from build123d import *

# Parameters (mm, degrees)
MODEL_R             = 4.950133
MODEL_R_2           = 1.45002
MODEL_R_3           = 1.45
MODEL_R_4           = 1.5
MODEL_W             = 4
MODEL_H             = 3
MODEL_W_2           = 21.736231
MODEL_W_3           = 3
MODEL_H_2           = 2
MODEL_W_4           = 2
MODEL_H_3           = 5
BOSS_EXTRUDE1_DEPTH = 3


with BuildPart() as part:
    # Model → Boss-Extrude1 (new body)
    with BuildSketch(Plane.XY):
        with BuildLine():
            Line((330.563429791, 166.163919592), (330.563429791, 120.063919592))
            Line((330.563429791, 120.063919592), (328.431544791, 120.063919592))
            Line((328.431544791, 120.063919592), (328.431544791, 117.063919592))
            Line((328.431544791, 117.063919592), (325.431544791, 117.063919592))
            Line((325.431544791, 117.063919592), (325.431544791, 120.063919592))
            Line((325.431544791, 120.063919592), (271.695313791, 120.063919592))
            Line((271.695313791, 120.063919592), (271.695313791, 117.063919592))
            Line((271.695313791, 117.063919592), (268.695313791, 117.063919592))
            Line((268.695313791, 117.063919592), (268.695313791, 120.063919592))
            Line((268.695313791, 120.063919592), (266.463429791, 120.063919592))
            Line((266.463429791, 120.063919592), (266.463429791, 122.295819592))
            Line((266.463429791, 122.295819592), (263.463429791, 122.295819592))
            Line((263.463429791, 122.295819592), (263.463429791, 125.295819592))
            Line((263.463429791, 125.295819592), (266.463429791, 125.295819592))
            Line((266.463429791, 125.295819592), (266.463429791, 154.799800566))
            ThreePointArc((266.463429791, 154.799800566), (267.463429791, 155.799800566), (266.463429791, 156.799800566))
            Line((266.463429791, 156.799800566), (266.463429791, 157.915840878))
            ThreePointArc((266.463429791, 157.915840878), (267.463429791, 158.915840878), (266.463429791, 159.915840878))
            Line((266.463429791, 159.915840878), (266.463429791, 160.932019592))
            Line((266.463429791, 160.932019592), (263.463429791, 160.932019592))
            Line((263.463429791, 160.932019592), (263.463429791, 163.932019592))
            Line((263.463429791, 163.932019592), (266.463429791, 163.932019592))
            Line((266.463429791, 163.932019592), (266.463429791, 166.163919592))
            Line((266.463429791, 166.163919592), (268.695313791, 166.163919592))
            Line((268.695313791, 166.163919592), (268.695313791, 169.163919592))
            Line((268.695313791, 169.163919592), (271.695313791, 169.163919592))
            Line((271.695313791, 169.163919592), (271.695313791, 166.163919592))
            Line((271.695313791, 166.163919592), (325.431544791, 166.163919592))
            Line((325.431544791, 166.163919592), (325.431544791, 169.163919592))
            Line((325.431544791, 169.163919592), (328.431544791, 169.163919592))
            Line((328.431544791, 169.163919592), (328.431544791, 166.163919592))
            Line((328.431544791, 166.163919592), (330.563429791, 166.163919592))
        make_face()
        with Locations((280.563429657, 143.113919537)):
            Circle(MODEL_R, mode=Mode.SUBTRACT)
        with Locations((280.563429791, 151.113919592)):
            Circle(MODEL_R_2, mode=Mode.SUBTRACT)
        with Locations((280.563429791, 135.113919592)):
            Circle(MODEL_R_3, mode=Mode.SUBTRACT)
        with Locations((315.431544791, 159.663919592)):
            Circle(MODEL_R_4, mode=Mode.SUBTRACT)
        with Locations((281.695313791, 159.663919592)):
            Circle(MODEL_R_4, mode=Mode.SUBTRACT)
        with Locations((315.431544791, 126.563919592)):
            Circle(MODEL_R_4, mode=Mode.SUBTRACT)
        with Locations((281.695313791, 126.563919592)):
            Circle(MODEL_R_4, mode=Mode.SUBTRACT)
        with Locations((311.663429791, 143.113919592)):
            Circle(MODEL_R_4, mode=Mode.SUBTRACT)
        with Locations((297.116645225, 144.3593347)):
            Circle(MODEL_R_4, mode=Mode.SUBTRACT)
        with Locations((273.695313791, 159.663919592)):
            Rectangle(MODEL_W, MODEL_H, mode=Mode.SUBTRACT)
        with Locations((298.563429291, 159.663919592)):
            Rectangle(MODEL_W_2, MODEL_H, mode=Mode.SUBTRACT)
        with Locations((323.431544791, 159.663919592)):
            Rectangle(MODEL_W, MODEL_H, mode=Mode.SUBTRACT)
        with Locations((273.695313791, 126.563919592)):
            Rectangle(MODEL_W, MODEL_H, mode=Mode.SUBTRACT)
        with Locations((298.563429291, 126.563919592)):
            Rectangle(MODEL_W_2, MODEL_H, mode=Mode.SUBTRACT)
        with Locations((323.431544791, 126.563919592)):
            Rectangle(MODEL_W, MODEL_H, mode=Mode.SUBTRACT)
        with Locations((314.063465132, 147.705010706)):
            Rectangle(MODEL_W_3, MODEL_H_2, mode=Mode.SUBTRACT)
        with Locations((308.063465132, 147.705010706)):
            Rectangle(MODEL_W_3, MODEL_H_2, mode=Mode.SUBTRACT)
        with Locations((314.063465132, 138.522828477)):
            Rectangle(MODEL_W_3, MODEL_H_2, mode=Mode.SUBTRACT)
        with Locations((308.063465132, 138.522828477)):
            Rectangle(MODEL_W_3, MODEL_H_2, mode=Mode.SUBTRACT)
        with Locations((327.563465132, 150.663919592)):
            Rectangle(MODEL_W_4, MODEL_H_3, mode=Mode.SUBTRACT)
        with Locations((327.563465132, 143.113919592)):
            Rectangle(MODEL_W_4, MODEL_H_3, mode=Mode.SUBTRACT)
        with Locations((327.563465132, 135.563919592)):
            Rectangle(MODEL_W_4, MODEL_H_3, mode=Mode.SUBTRACT)
        with BuildLine():
            ThreePointArc((275.146294982, 151.69745945), (272.799630894, 149.651957033), (271.18327611, 146.991447741))
            ThreePointArc((271.18327611, 146.991447741), (271.860939302, 145.358728353), (273.49365869, 146.036391545))
            ThreePointArc((273.49365869, 146.036391545), (274.711896566, 148.041603035), (276.48056463, 149.583287152))
            ThreePointArc((276.48056463, 149.583287152), (276.870515955, 151.307508126), (275.146294982, 151.69745945))
        make_face(mode=Mode.SUBTRACT)
        with BuildLine():
            ThreePointArc((271.183276501, 139.236391494), (272.799631045, 136.575882517), (275.146294756, 134.530380266))
            ThreePointArc((275.146294756, 134.530380266), (276.870515729, 134.92033159), (276.480564405, 136.644552563))
            ThreePointArc((276.480564405, 136.644552563), (274.711896718, 138.186236515), (273.493659081, 140.191447689))
            ThreePointArc((273.493659081, 140.191447689), (271.860939693, 140.869110881), (271.183276501, 139.236391494))
        make_face(mode=Mode.SUBTRACT)
        with BuildLine():
            ThreePointArc((289.943583204, 146.991447741), (288.327228421, 149.651957033), (285.980564333, 151.69745945))
            ThreePointArc((285.980564333, 151.69745945), (284.25634336, 151.307508126), (284.646294684, 149.583287152))
            ThreePointArc((284.646294684, 149.583287152), (286.414962749, 148.041603035), (287.633200625, 146.036391545))
            ThreePointArc((287.633200625, 146.036391545), (289.265920012, 145.358728353), (289.943583204, 146.991447741))
        make_face(mode=Mode.SUBTRACT)
        with BuildLine():
            ThreePointArc((284.64629491, 136.644552563), (286.414962597, 138.186236515), (287.633200234, 140.191447689))
            ThreePointArc((287.633200234, 140.191447689), (289.265919735, 140.869110884), (289.94358293, 139.236391383))
            ThreePointArc((289.94358293, 139.236391383), (288.327228286, 136.575882304), (285.980564432, 134.530380008))
            ThreePointArc((285.980564432, 134.530380008), (284.256343393, 134.920331525), (284.64629491, 136.644552563))
        make_face(mode=Mode.SUBTRACT)
    extrude(amount=BOSS_EXTRUDE1_DEPTH)


solid = part.part
Here's how the part is built. I have some questions about the finished solid (model axes, mm). A direction names the side the tool comes from. Coordinates: 2 decimals unless noted, no trailing zeros. Write each loop counter-clockwise with the first axis right and the second up, starting at its lowest first coordinate (ties: lowest second). Pieces come first, ordered by that corner, then holes.
Item 1: On a 3-axis mill with a long thin cutter (end or side, diameter ignored), from which of +Z, -Z, +X, -X, +Y, -Y can I reach the whole of each face in a straight line? I mean faces 1 (the flat face through (328, 153.164, 1)), 2 (the flat face through (265, 125.296, 1)), 3 (the flat face through (325.432, 119, 1)). Say none if no direction works.
Item 2: If I drill on line 1 (Y direction, x = 323, z = 0.7); line 2 (Y direction, x = 279.5, z = 1.8); line 3 (Y direction, x = 276.5, z = 0.3), over which ranges is the centre line in solid material (lowest first)?
Item 3: I want a section at C-C on y = 129.5. Write out the boundary of the cut face in (x, z), and give its area (3 significant figures).
Item 4: I want a section at A-A on x = 303. Write out the boundary of the cut face in (y, z), and give its area (3 significant figures).
Item 5: If we mould it in two halves opening along Y, with no side actions, what happens to faces 4 (the flat face through (263.463, 162, 1)), 5 (the flat face through (275.695, 127, 1)), 6 (the flat face through (268, 166.164, 1))? For each: +Y half, -Y half, draft (parallel to the pull), parting line (faces both ways), or undercut.
Item 6: I want a section at B-B on x = 281. Write out the boundary of the cut face in (y, z), and give its area (3 significant figures).
Item 7: Will these pins go through, and if not, where does the flat tip stop? pin 1 (1.5 mm diameter, centred on y = 142, z = 1, fed in from -X); pin 2 (1.5 mm diameter, centred on x = 308, z = 1, fed in from -Y); pin 3 (2.5 mm diameter, centred on x = 315.43, y = 126.56, fed in from -Z).
Item 8: I want a section at D-D on z = 0.95. Count the separate pieces of the cut face and the enclosed holes in it, and give its area (3 significant figures).
Findings below:
1. face 1: +Z, -Z
1. face 2: +Z, -Z, -X
1. face 3: +Z, -Z, -Y
2. line 1: y = 120.06 to 125.06, 128.06 to 158.16, 161.16 to 166.16
2. line 2: y = 120.06 to 134.13, 136.1 to 138.28, 147.95 to 150.13, 152.1 to 166.16
2. line 3: y = 120.06 to 134.54, 136.63 to 140.29, 145.94 to 149.6, 151.68 to 166.16
3. outline: (266.46, 0) - (330.56, 0) - (330.56, 3) - (266.46, 3) - close
3. area: 192 mm2
4. outline: (120.06, 0) - (125.06, 0) - (125.06, 3) - (120.06, 3) - close; (128.06, 0) - (158.16, 0) - (158.16, 3) - (128.06, 3) - close; (161.16, 0) - (166.16, 0) - (166.16, 3) - (161.16, 3) - close
4. area: 120 mm2
5. face 4: draft
5. face 5: undercut
5. face 6: +Y half
6. outline: (120.06, 0) - (125.23, 0) - (125.23, 3) - (120.06, 3) - close; (127.89, 0) - (133.73, 0) - (133.73, 3) - (127.89, 3) - close; (136.5, 0) - (138.18, 0) - (138.18, 3) - (136.5, 3) - close; (148.04, 0) - (149.73, 0) - (149.73, 3) - (148.04, 3) - close; (152.5, 0) - (158.33, 0) - (158.33, 3) - (152.5, 3) - close; (160.99, 0) - (166.16, 0) - (166.16, 3) - (160.99, 3) - close
6. area: 76.2 mm2
7. pin 1: stops at x = 266.46
7. pin 2: stops at y = 120.06
7. pin 3: passes through
8. separate pieces: 1
8. enclosed holes: 26
8. area: 2,570 mm2
